Verification items for this drawing (mm, ordinates from the low corner). Coordinates: 2 decimals unless noted, no trailing zeros. Loops run counter-clockwise (first coordinate to the right, second up) from the corner with the lowest first, then second, coordinate; pieces in that order, holes last. Notation, with made-up numbers: M 84,-30 L 109,-30 A24 cw 109,-14 Z; hole C 21.25,-21 d1. An arc over 180 degrees is marked long. One line per question, with ' | ' between items. Start each with the question number.
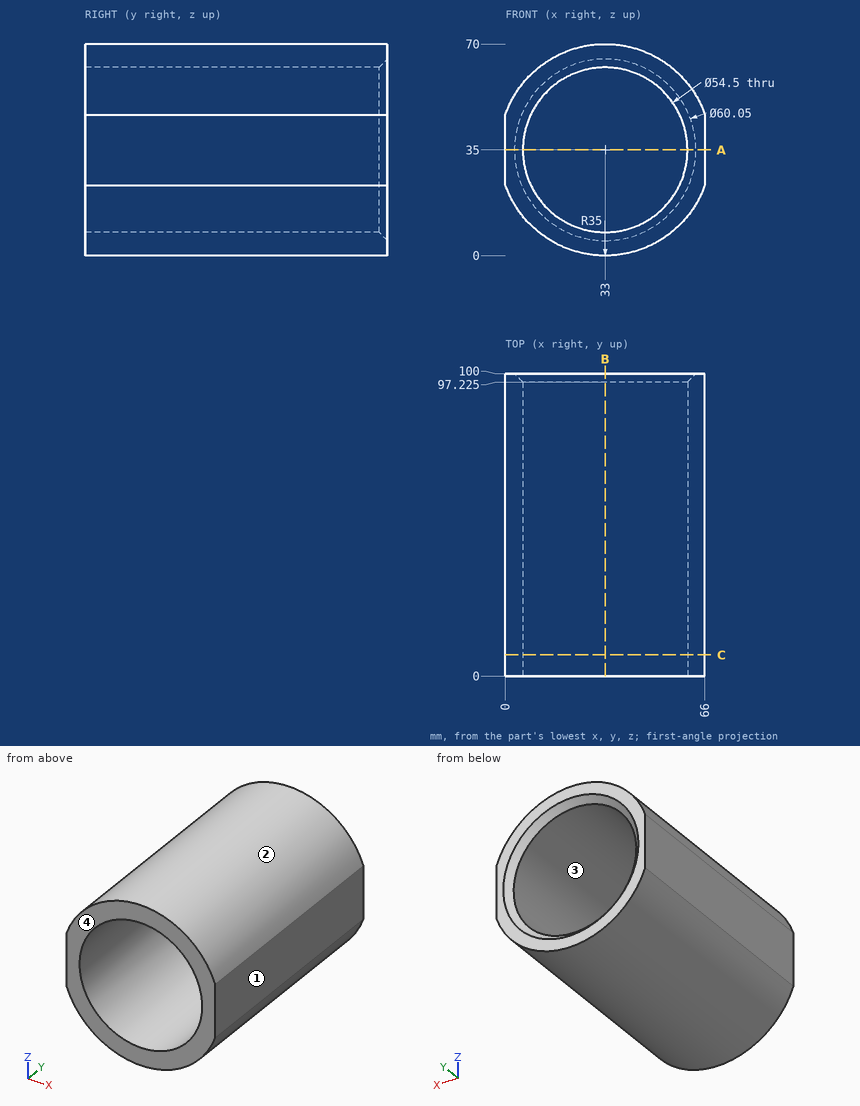
1. Sectioned sample at A-A (z = 35). Record the cut outline in (x, y) (3 decimals).
2. Draft check along X on the marked faces 1, 2, 3 and 4. Enter one of: +X half, -X half, draft (parallel to the pull), parting line (faces both ways), or undercut.
3. Sectioned sample at B-B (x = 33). Record the cut outline in (y, z) (3 decimals), and give its area (3 significant figures).
4. Sectioned sample at C-C (y = 7). Record the cut outline in (x, z).
5. Thickness scan on line 1 (Z direction, x = 33, y = 74); line 2 (X direction, y = 47, z = 35); line 3 (X direction, y = 86, z = 28). Record the ranges inside material, lowest first.
6. Depth check by flat-ended pin: pin 1 Ø8 at (x, y) = (51, 17) entering from +Z; pin 2 Ø2 at (x, y) = (43, 31) entering from -Z; pin 3 Ø8 at (y, z) = (34, 11.5) entering from +X. Enter the tip coordinate at first touch or a pass-through.
Result:
1) outline: M 0,0 L 5.75,0 L 5.75,97.225 L 2.975,100 L 0,100 Z; M 60.25,0 L 66,0 L 66,100 L 63.025,100 L 60.25,97.225 Z
2) face 1: +X half | face 2: parting line | face 3: undercut | face 4: draft
3) outline: M 0,0 L 100,0 L 100,4.975 L 97.225,7.75 L 0,7.75 Z; M 0,62.25 L 97.225,62.25 L 100,65.025 L 100,70 L 0,70 Z | area: 1,540 mm2
4) outline: M 0,23.34 A35 ccw 66,23.34 L 66,46.66 A35 ccw 0,46.66 Z; hole C 33,35 d54.5
5) line 1: z = 0 to 7.75, 62.25 to 70 | line 2: x = 0 to 5.75, 60.25 to 66 | line 3: x = 0 to 6.66, 59.34 to 66
6) pin 1: stops at z = 67.08 | pin 2: stops at z = 1.18 | pin 3: stops at x = 62.06
